from build123d import *

# Parameters (mm, degrees)
F0_R     = 2
F0_R_2   = 21
F1_DEPTH = 5


with BuildPart() as f1:
    # F0 (on Front) → F1 (new body)
    with BuildSketch(Plane.XZ):
        with BuildLine():
            ThreePointArc((-25.119935, 34.380065), (-32.949747, 32.949747), (-34.380065, 25.119935))
            Line((-34.380065, 25.119935), (-30.309803, 16.103286))
            ThreePointArc((-30.309803, 16.103286), (-29.695207, 13.496561), (-30.104507, 10.849823))
            ThreePointArc((-30.104507, 10.849823), (-32, 0), (-30.104507, -10.849823))
            ThreePointArc((-30.104507, -10.849823), (-29.695207, -13.496561), (-30.309803, -16.103287))
            Line((-30.309803, -16.103287), (-34.380065, -25.119937))
            ThreePointArc((-34.380065, -25.119937), (-32.949747, -32.949749), (-25.119935, -34.380066))
            Line((-25.119935, -34.380066), (-16.103285, -30.309804))
            ThreePointArc((-16.103285, -30.309804), (-13.49656, -29.695207), (-10.849822, -30.104507))
            ThreePointArc((-10.849822, -30.104507), (1e-06, -32), (10.849823, -30.104507))
            ThreePointArc((10.849823, -30.104507), (13.496561, -29.695207), (16.103286, -30.309803))
            Line((16.103286, -30.309803), (25.119935, -34.380065))
            ThreePointArc((25.119935, -34.380065), (32.949747, -32.949747), (34.380065, -25.119935))
            Line((34.380065, -25.119935), (30.309803, -16.103286))
            ThreePointArc((30.309803, -16.103286), (29.695207, -13.496561), (30.104507, -10.849823))
            ThreePointArc((30.104507, -10.849823), (32, 0), (30.104507, 10.849823))
            ThreePointArc((30.104507, 10.849823), (29.695207, 13.496561), (30.309803, 16.103286))
            Line((30.309803, 16.103286), (34.380065, 25.119935))
            ThreePointArc((34.380065, 25.119935), (32.949747, 32.949747), (25.119935, 34.380065))
            Line((25.119935, 34.380065), (16.103286, 30.309803))
            ThreePointArc((16.103286, 30.309803), (13.496561, 29.695207), (10.849823, 30.104507))
            ThreePointArc((10.849823, 30.104507), (0, 32), (-10.849823, 30.104507))
            ThreePointArc((-10.849823, 30.104507), (-13.496561, 29.695207), (-16.103286, 30.309803))
            Line((-16.103286, 30.309803), (-25.119935, 34.380065))
        make_face()
        with Locations((-28, -28.000001)):
            Circle(F0_R, mode=Mode.SUBTRACT)
        with Locations((-22, -14.773287)):
            Circle(F0_R, mode=Mode.SUBTRACT)
        with Locations((28, -28)):
            Circle(F0_R, mode=Mode.SUBTRACT)
        with Locations((22, -14.773287)):
            Circle(F0_R, mode=Mode.SUBTRACT)
        with Locations((-19, 18.472953)):
            Circle(F0_R, mode=Mode.SUBTRACT)
        with Locations((-28, 28)):
            Circle(F0_R, mode=Mode.SUBTRACT)
        Circle(F0_R_2, mode=Mode.SUBTRACT)
        with Locations((19, 18.472953)):
            Circle(F0_R, mode=Mode.SUBTRACT)
        with Locations((28, 28)):
            Circle(F0_R, mode=Mode.SUBTRACT)
    extrude(amount=F1_DEPTH)


solid = f1.part
Geometry check sheet. Reference: the model listing, model coordinates, mm. A direction names the side the tool comes from. Coordinates: 2 decimals unless noted, no trailing zeros. Order: outer loops, then holes, each group sorted by start corner. A loop starts at its lowest first (then second) coordinate and runs counter-clockwise, first axis right, second up. Notation, with made-up numbers: (15, 12.25) - (45, 12.25) arc R17 cw to (45, 39.25) - close; hole circle Ø7 at (2.25, 52.25). An arc over 180 degrees is marked (long way). Answer in a Markdown table with one row per item. Add a question column.
1) Cross-section at A-A, the plane z = 0. Record the cut outline in (x, y), then the cut area to 3 significant figures.
2) Gauge pin test, flat ends, axial feed: P1, Ø1, axis at y = -3, z = 8, coming from the +X side; P2, Ø1, axis at x = 8.5, y = -1.5, coming from the +Z side; P3, Ø1, axis at y = -1, z = -13.5, coming from the -X side. Record the tip position at first contact, or that the pin passes through.
3) Material ranges on line 1 along Z through (x, y) = (-28, -1.9); line 2 along X through (y, z) = (-1.35, -26.5); line 3 along Z through (x, y) = (-29, -4), recorded low to high. Write a range as [from, to].
4) Set-up check for faces 1 (the flat face through (32.37, -2.46, -20.67)), 2 (the flat face through (-20.548, -2.465, 32.316)), 3 (the flat face through (-32.316, -2.465, -20.548)), 4 (the flat face through (20.548, -2.465, -32.316)): record each of +Z, -Z, +X, -X, +Y, -Y from which the full face is reachable in a straight line by a thin tool's end or side.
5) Release check for a two-part mould opening along Z. For faces 5 (the flat face through (32.316, -2.465, 20.548)), 6 (the flat face through (15, -5, -15)), 7 (the cylindrical face through (0, -2, 32)), 8 (the cylindrical face through (29.697, -2.465, -13.534)) record: +Z half, -Z half, draft (parallel to the pull), parting line (faces both ways), or undercut.
6) Cross-section at C-C, the plane y = -2.85. State how many separate pieces and enclosed holes the cut face has, then the cut area to 3 significant figures.
7) Cross-section at D-D, the plane x = -22. Record the cut outline in (y, z).
8) Cross-section at B-B, the plane x = 28. Record the cut outline in (y, z).
Check result:
| question | item | result |
|---|---|---|
| 1 | outline | (-32, -5) - (-21, -5) - (-21, 0) - (-32, 0) - close; (21, -5) - (32, -5) - (32, 0) - (21, 0) - close |
| 1 | area | 110 mm² |
| 2 | P1 | stops at x = 31.11 |
| 2 | P2 | stops at z = 30.98 |
| 2 | P3 | stops at x = -29.73 |
| 3 | line 1 | z = [-35, -30], [-26, 26], [30, 35] |
| 3 | line 2 | x = [-34.84, -29.32], [-26.68, 26.68], [29.32, 34.84] |
| 3 | line 3 | z = [-34.93, -29.73], [-26.27, 26.27], [29.73, 34.93] |
| 4 | face 1 | +X, +Y, -Y |
| 4 | face 2 | +Z, +Y, -Y |
| 4 | face 3 | -X, +Y, -Y |
| 4 | face 4 | -Z, +Y, -Y |
| 5 | face 5 | undercut |
| 5 | face 6 | draft |
| 5 | face 7 | +Z half |
| 5 | face 8 | undercut |
| 6 | separate pieces | 1 |
| 6 | enclosed holes | 9 |
| 6 | area | 2,650 mm² |
| 7 | outline | (-5, -32.97) - (0, -32.97) - (0, -16.77) - (-5, -16.77) - close; (-5, -12.77) - (0, -12.77) - (0, 32.97) - (-5, 32.97) - close |
| 8 | outline | (-5, -35) - (0, -35) - (0, -30) - (-5, -30) - close; (-5, -26) - (0, -26) - (0, 26) - (-5, 26) - close; (-5, 30) - (0, 30) - (0, 35) - (-5, 35) - close |
